CAD build for the part. Positions are in the model's coordinates, mm. Round coordinates to 2 decimals unless told otherwise and drop trailing zeros. Order: outer loops, then holes, each group sorted by start corner. A loop starts at its lowest first (then second) coordinate and runs counter-clockwise, first axis right, second up. Notation, with made-up numbers: (37.25, 14.25) -> (64.25, 14.25) arc R29 ccw to (64.25, 51.25) -> close; hole circle Ø6 at (40, -6.5). An arc over 180 degrees is marked (long way). Return JSON: item names as keys, results as strings. Group by question number.
Q1. Cut at D-D (y = -126). Write the cut outline in (x, z), then the cut area to 3 significant figures.
Q2. Probe line 1 along Z through (x, y) = (0.8, 0); line 2 along Y through (x, z) = (0.8, 99); line 3 along Y through (x, z) = (0.4, 61.5). List the from-to ranges inside material, lowest first.
Q3. Cut at B-B (z = 42). Write the cut outline in (x, y).
Q4. Flat gauge pins, fed straight in: pin 1 (0.5 mm diameter, centred on x = 1, y = 0, fed in from +Z); pin 2 (0.5 mm diameter, centred on x = 0.5, y = 0.5, fed in from +Z); pin 3 (0.5 mm diameter, centred on x = 0.5, y = 0.5, fed in from -Z); pin 4 (2 mm diameter, centred on y = -98, z = 131.5, fed in from -X). Where does each tip first touch, or does it go through?
Q5. Cut at A-A (y = -14). Write the cut outline in (x, z), then the cut area to 3 significant figures.
Q6. Cut at C-C (x = 1.2). Count the separate pieces of the cut face and the enclosed holes in it, then the cut area to 3 significant figures.
Autodesk Inventor part; units mm, degrees
ref_plane "YZ Plane" through (0, 0, 0) normal (1, 0, 0) x (0, 1, 0)
ref_plane "XZ Plane" through (0, 0, 0) normal (0, 1, 0) x (-1, 0, 0)
ref_plane "XY Plane" through (0, 0, 0) normal (0, 0, 1) x (1, 0, 0)
sketch "main" plane through (0, 0, 0) normal (0, 0, 1) x (1, 0, 0)
  circle A0 centre (2982.9462, -106.4126) radius 2.1844
  circle A1 centre (2838.6663, 17.9802) radius 2.1844
  arc A2 (2982.9462, -187.3751) -> (2987.7082, -182.5494) centre (2982.9462, -182.6126) ccw
  arc A3 (2987.7082, -106.4758) -> (2986.0859, -102.8316) centre (2982.9462, -106.4126) ccw
  arc A4 (2842.8526, 22.7548) -> (2833.5352, 14.2393) centre (2838.6663, 17.9802) ccw
  line L0 (2987.7082, -106.4758) -> (2987.7082, -182.5494)
  line L1 (2986.0859, -102.8316) -> (2842.8526, 22.7548)
  line L2 (2981.1428, -180.3012) -> (2984.7496, -180.3012)
  line L3 (2985.2576, -180.8092) -> (2985.2576, -184.416)
  line L4 (2984.7496, -184.924) -> (2981.1428, -184.924)
  line L5 (2980.6348, -184.416) -> (2980.6348, -180.8092)
  line L6 (2980.6348, -180.3012) -> (2985.2576, -184.924) construction
  line L7 (2985.2576, -180.3012) -> (2980.6348, -184.924) construction
  line L8 (2981.1428, -167.6012) -> (2984.7496, -167.6012)
  line L9 (2985.2576, -168.1092) -> (2985.2576, -171.716)
  line L10 (2984.7496, -172.224) -> (2981.1428, -172.224)
  line L11 (2980.6348, -171.716) -> (2980.6348, -168.1092)
  line L12 (2980.6348, -167.6012) -> (2985.2576, -172.224) construction
  line L13 (2985.2576, -167.6012) -> (2980.6348, -172.224) construction
  line L14 (2981.1428, -154.9012) -> (2984.7496, -154.9012)
  line L15 (2985.2576, -155.4092) -> (2985.2576, -159.016)
  line L16 (2984.7496, -159.524) -> (2981.1428, -159.524)
  line L17 (2980.6348, -159.016) -> (2980.6348, -155.4092)
  line L18 (2980.6348, -154.9012) -> (2985.2576, -159.524) construction
  line L19 (2985.2576, -154.9012) -> (2980.6348, -159.524) construction
  arc A5 (2984.7496, -184.924) -> (2985.2576, -184.416) centre (2984.7496, -184.416) ccw
  arc A6 (2980.6348, -184.416) -> (2981.1428, -184.924) centre (2981.1428, -184.416) ccw
  arc A7 (2981.1428, -180.3012) -> (2980.6348, -180.8092) centre (2981.1428, -180.8092) ccw
  arc A8 (2985.2576, -180.8092) -> (2984.7496, -180.3012) centre (2984.7496, -180.8092) ccw
  arc A9 (2984.7496, -172.224) -> (2985.2576, -171.716) centre (2984.7496, -171.716) ccw
  arc A10 (2980.6348, -171.716) -> (2981.1428, -172.224) centre (2981.1428, -171.716) ccw
  arc A11 (2981.1428, -167.6012) -> (2980.6348, -168.1092) centre (2981.1428, -168.1092) ccw
  arc A12 (2985.2576, -168.1092) -> (2984.7496, -167.6012) centre (2984.7496, -168.1092) ccw
  arc A13 (2984.7496, -159.524) -> (2985.2576, -159.016) centre (2984.7496, -159.016) ccw
  arc A14 (2980.6348, -159.016) -> (2981.1428, -159.524) centre (2981.1428, -159.016) ccw
  arc A15 (2981.1428, -154.9012) -> (2980.6348, -155.4092) centre (2981.1428, -155.4092) ccw
  arc A16 (2985.2576, -155.4092) -> (2984.7496, -154.9012) centre (2984.7496, -155.4092) ccw
  line L20 (2982.9462, -187.3751) -> (2978.2364, -187.3751)
  line L21 (2975.647, -186.0374) -> (2833.5352, 14.2393)
  arc A17 (2975.647, -186.0374) -> (2978.2364, -187.3751) centre (2978.2364, -184.2001) ccw
  line L22 (2961.0316, -101.9771) -> (2893.3678, -42.6497)
  line L23 (2971.8332, -117.8521) -> (2971.8332, -153.2302)
  line L24 (2961.0316, -101.9771) -> (2935.4651, -101.9771)
  line L25 (2971.8332, -117.8521) -> (2946.7297, -117.8521)
  line L26 (2893.3678, -42.6497) -> (2935.4651, -101.9771)
  line L27 (2946.7297, -117.8521) -> (2971.8332, -153.2302)
  point P0 (2935.9211, -90.1281)
  point P1 (2982.9462, -169.9126)
  point P2 (2982.9462, -157.2126)
  point P3 (2976.5962, -187.3751)
  point P4 (2959.2815, -117.8521)
  dimension "d0" = 12.7
  dimension "d1" = 9.525
  dimension "d2" = 9.525
  dimension "d7" = 4.6228
  dimension "d8" = 4.6228
  dimension "d9" = 4.6228
  dimension "d10" = 4.6228
  dimension "d11" = 4.6228
  dimension "d12" = 4.6228
  dimension "d13" = 0.508
  dimension "d14" = 6.35
  dimension "d15" = 3.175
  dimension "d18" = 15.875
  dimension "d19" = 15.875
  dimension "d20" = 15.875
  dimension "d21" = 15.875
  dimension "d22" = 15.875
sketch "Sketch1" plane through (0, 0, 0) normal (1, 0, 0) x (0, 1, 0)
  circle A0 centre (0, 76.2) radius 2.1844
  circle A1 centre (-144.2799, 200.5928) radius 2.1844
  arc A2 (0, -4.7625) -> (4.7621, 0.0632) centre (0, 0) ccw
  arc A3 (4.7621, 76.1368) -> (3.1398, 79.781) centre (0, 76.2) ccw
  arc A4 (-140.0936, 205.3674) -> (-149.411, 196.8519) centre (-144.2799, 200.5928) ccw
  line L0 (4.7621, 76.1368) -> (4.7621, 0.0632)
  line L1 (3.1398, 79.781) -> (-140.0936, 205.3674)
  line L2 (-1.8034, 2.3114) -> (1.8034, 2.3114)
  line L3 (2.3114, 1.8034) -> (2.3114, -1.8034)
  line L4 (1.8034, -2.3114) -> (-1.8034, -2.3114)
  line L5 (-2.3114, -1.8034) -> (-2.3114, 1.8034)
  line L6 (-2.3114, 2.3114) -> (2.3114, -2.3114) construction
  line L7 (2.3114, 2.3114) -> (-2.3114, -2.3114) construction
  line L8 (-1.8034, 15.0114) -> (1.8034, 15.0114)
  line L9 (2.3114, 14.5034) -> (2.3114, 10.8966)
  line L10 (1.8034, 10.3886) -> (-1.8034, 10.3886)
  line L11 (-2.3114, 10.8966) -> (-2.3114, 14.5034)
  line L12 (-2.3114, 15.0114) -> (2.3114, 10.3886) construction
  line L13 (2.3114, 15.0114) -> (-2.3114, 10.3886) construction
  line L14 (-1.8034, 27.7114) -> (1.8034, 27.7114)
  line L15 (2.3114, 27.2034) -> (2.3114, 23.5966)
  line L16 (1.8034, 23.0886) -> (-1.8034, 23.0886)
  line L17 (-2.3114, 23.5966) -> (-2.3114, 27.2034)
  line L18 (-2.3114, 27.7114) -> (2.3114, 23.0886) construction
  line L19 (2.3114, 27.7114) -> (-2.3114, 23.0886) construction
  arc A5 (1.8034, -2.3114) -> (2.3114, -1.8034) centre (1.8034, -1.8034) ccw
  arc A6 (-2.3114, -1.8034) -> (-1.8034, -2.3114) centre (-1.8034, -1.8034) ccw
  arc A7 (-1.8034, 2.3114) -> (-2.3114, 1.8034) centre (-1.8034, 1.8034) ccw
  arc A8 (2.3114, 1.8034) -> (1.8034, 2.3114) centre (1.8034, 1.8034) ccw
  arc A9 (1.8034, 10.3886) -> (2.3114, 10.8966) centre (1.8034, 10.8966) ccw
  arc A10 (-2.3114, 10.8966) -> (-1.8034, 10.3886) centre (-1.8034, 10.8966) ccw
  arc A11 (-1.8034, 15.0114) -> (-2.3114, 14.5034) centre (-1.8034, 14.5034) ccw
  arc A12 (2.3114, 14.5034) -> (1.8034, 15.0114) centre (1.8034, 14.5034) ccw
  arc A13 (1.8034, 23.0886) -> (2.3114, 23.5966) centre (1.8034, 23.5966) ccw
  arc A14 (-2.3114, 23.5966) -> (-1.8034, 23.0886) centre (-1.8034, 23.5966) ccw
  arc A15 (-1.8034, 27.7114) -> (-2.3114, 27.2034) centre (-1.8034, 27.2034) ccw
  arc A16 (2.3114, 27.2034) -> (1.8034, 27.7114) centre (1.8034, 27.2034) ccw
  line L20 (0, -4.7625) -> (-4.7098, -4.7625)
  line L21 (-7.2992, -3.4248) -> (-149.411, 196.8519)
  arc A17 (-7.2992, -3.4248) -> (-4.7098, -4.7625) centre (-4.7098, -1.5875) ccw
  line L22 (-21.9146, 80.6355) -> (-89.5784, 139.9629)
  line L23 (-11.1129, 64.7605) -> (-11.1129, 29.3823)
  line L24 (-21.9146, 80.6355) -> (-47.481, 80.6355)
  line L25 (-11.1129, 64.7605) -> (-36.2165, 64.7605)
  line L26 (-89.5784, 139.9629) -> (-47.481, 80.6355)
  line L27 (-36.2165, 64.7605) -> (-11.1129, 29.3823)
extrude "Extrusion1" add sketch "Sketch1" along normal blind 1.5875
properties part number "Triiangle Gusset" material "Acetal Resin, White"
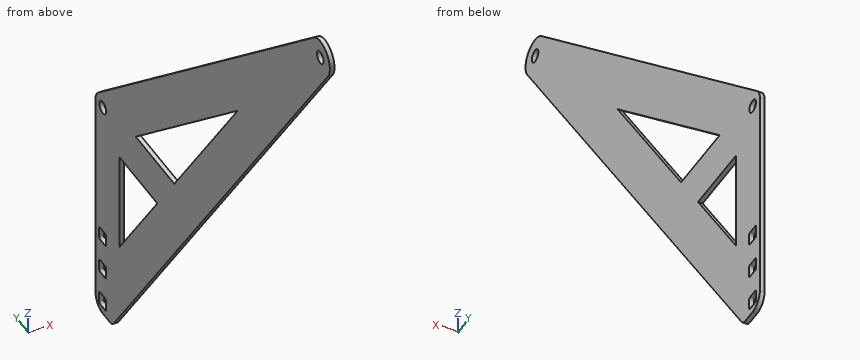
Solution:
{
 "1": {"outline": "(0, 163.86) -> (1.59, 163.86) -> (1.59, 193.01) -> (0, 193.01) -> close", "area": "46.3 mm²"},
 "2": {"line 1": "z = -4.76 to -2.31, 2.31 to 10.39, 15.01 to 23.09, 27.71 to 74.02, 78.38 to 82.53", "line 2": "y = -79.98 to -60.51, -42.86 to -18.78", "line 3": "y = -53.37 to -33.9, -11.11 to 4.76"},
 "3": {"outline": "(0, -39.53) -> (1.59, -39.53) -> (1.59, -20.07) -> (0, -20.07) -> close; (0, -11.11) -> (1.59, -11.11) -> (1.59, 4.76) -> (0, 4.76) -> close"},
 "4": {"pin 1": "stops at z = 82.75", "pin 2": "stops at z = 82.31", "pin 3": "stops at z = -4.76", "pin 4": "stops at x = 0"},
 "5": {"outline": "(0, 6.02) -> (1.59, 6.02) -> (1.59, 33.45) -> (0, 33.45) -> close; (0, 64.76) -> (1.59, 64.76) -> (1.59, 94.81) -> (0, 94.81) -> close", "area": "91.3 mm²"},
 "6": {"separate pieces": "1", "enclosed holes": "7", "area": "7,490 mm²"}
}
